Print and shaded views of the part. All mm, measured from the part's lowest x, y and z. A direction names the side the tool comes from. Give positions to 0.01 mm unless a question says otherwise; leave off trailing zeros. Order: outer loops, then holes, each group sorted by start corner. A loop starts at its lowest first (then second) coordinate and runs counter-clockwise, first axis right, second up. Notation, with made-up numbers: (43, 62) - (51, 62) arc R12 ccw to (51, 76) - close; hole circle Ø8 at (-8, -36). An arc over 180 degrees is marked (long way). Answer in a Markdown table with one row per item.
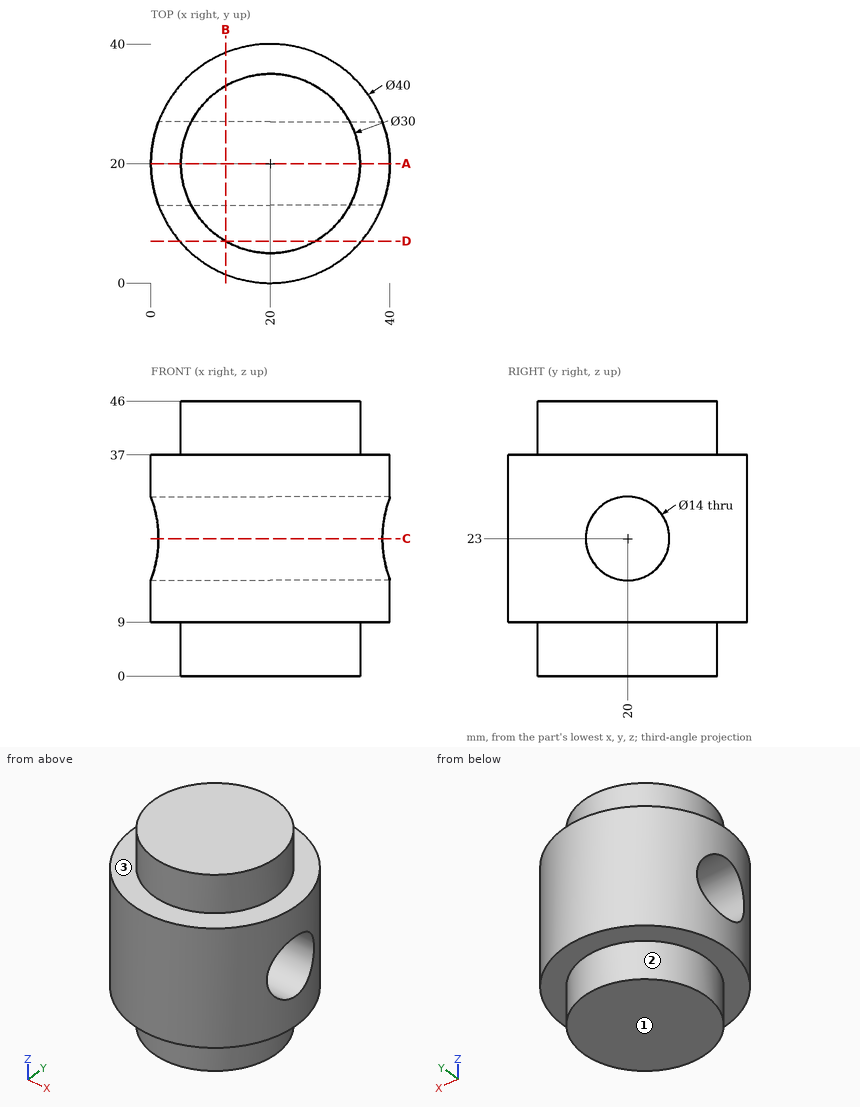
1. Cut at C-C on z = 23. Write the cut outline in (x, y) (3 decimals).
Check result:
| item | result |
|---|---|
| outline | (1.265, 13) arc R20 ccw to (38.735, 13) - close; (1.265, 27) - (38.735, 27) arc R20 ccw to start |
2. Cut at A-A on y = 20. Write the cut outline in (x, z).
Check result:
| item | result |
|---|---|
| outline | (0, 9) - (5, 9) - (5, 0) - (35, 0) - (35, 9) - (40, 9) - (40, 16) - (0, 16) - close; (0, 30) - (40, 30) - (40, 37) - (35, 37) - (35, 46) - (5, 46) - (5, 37) - (0, 37) - close |
3. Probe line 1 (Z direction, x = 30, y = 20); line 2 (Z direction, x = 26, y = 2); line 3 (Y direction, x = 33.5, z = 23). List the from-to ranges inside material, lowest first.
Check result:
| item | result |
|---|---|
| line 1 | z = 0 to 16, 30 to 46 |
| line 2 | z = 9 to 37 |
| line 3 | y = 5.24 to 13, 27 to 34.76 |
4. Which spindle directions (+Z, -Z, +X, -X, +Y, -Y) get a long thin tool onto all of the face, cutting with end or side? Do the marked faces 1, 2 and 3. Say none if no direction does.
Check result:
| item | result |
|---|---|
| face 1 | -Z, +X, -X, +Y, -Y |
| face 2 | -Z |
| face 3 | +Z |
5. Cut at D-D on y = 7. Write the cut outline in (x, z).
Check result:
| item | result |
|---|---|
| outline | (4.8, 9) - (12.52, 9) - (12.52, 0) - (27.48, 0) - (27.48, 9) - (35.2, 9) - (35.2, 37) - (27.48, 37) - (27.48, 46) - (12.52, 46) - (12.52, 37) - (4.8, 37) - close |
6. Drop flat-ended pins along their axis: P1, Ø5, axis at y = 12.5, z = 18.5, coming from the -X side; P2, Ø5, axis at x = 30.5, z = 25, coming from the +Y side; P3, Ø1, axis at x = 19, z = 35, coming from the +Y side; P4, Ø11, axis at y = 20, z = 23, coming from the +X side. Give the stop position or say it passes through.
Check result:
| item | result |
|---|---|
| P1 | stops at x = 0.64 |
| P2 | stops at y = 38.33 |
| P3 | stops at y = 39.99 |
| P4 | passes through |
7. Cut at B-B on x = 12.5. Write the cut outline in (y, z).
Check result:
| item | result |
|---|---|
| outline | (1.46, 9) - (7.01, 9) - (7.01, 0) - (32.99, 0) - (32.99, 9) - (38.54, 9) - (38.54, 37) - (32.99, 37) - (32.99, 46) - (7.01, 46) - (7.01, 37) - (1.46, 37) - close; hole circle Ø14 at (20, 23) |
